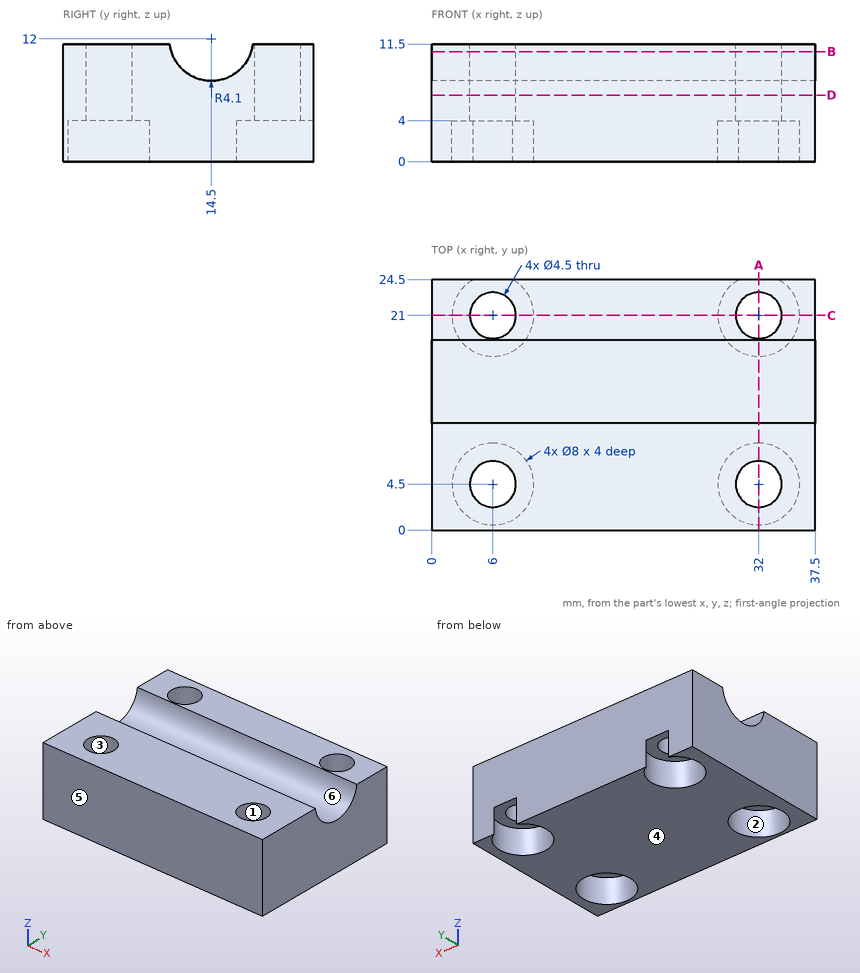
The drawing under review shows one solid part. Ordinate dimensions are in mm from its lowest x, y, z. A direction names the side the tool comes from. Round coordinates to 2 decimals unless told otherwise and drop trailing zeros. Order: outer loops, then holes, each group sorted by start corner. A loop starts at its lowest first (then second) coordinate and runs counter-clockwise, first axis right, second up. Notation, with made-up numbers: M -19,81.25 L -6,81.25 A26 cw -6,116.25 Z; hole C 3.25,12 d4. An arc over 180 degrees is marked long. Answer as CSV lines item,"result". Start each with the question number.
1) For pin 1 Ø3.5 at (x, y) = (6, 21) entering from +Z; pin 2 Ø4 at (x, y) = (6.5, 4) entering from -Z, all flat-tipped, find the tip position at first contact; note any pin that passes through.
2) Tool access review of the marked faces 1 and 2: name each direction out of +Z, -Z, +X, -X, +Y, -Y from which nothing blocks a thin tool from reaching the whole face with its end or side.
3) Add section C-C (y = 21). Give the boundary of the cut face in (x, z), then the cut area to 3 significant figures.
4) The part is to be moulded in two halves that separate along Y. For the marked faces 3, 4, 5 and 6, say which applies: +Y half, -Y half, draft (parallel to the pull), parting line (faces both ways), or undercut.
5) Wall thickness on line 1 along X through (y, z) = (4.5, 5.5); line 2 along X through (y, z) = (4.5, 2.8); line 3 along Y through (x, z) = (6, 8.5): over which ranges is each line inside the solid? List them lowest first. Write a range as [from, to].
6) Add section A-A (x = 32). Give the boundary of the cut face in (y, z), then the cut area to 3 significant figures.
7) Add section B-B (z = 10.75). Give the boundary of the cut face in (x, y).
8) Add section D-D (z = 6.5). Give the boundary of the cut face in (x, y), then the cut area to 3 significant figures.
Resolved:
1,pin 1,"through"
1,pin 2,"z = 4"
2,face 1,"+Z, -Z"
2,face 2,"-Z"
3,outline,"M 0,0 L 2,0 L 2,4 L 3.75,4 L 3.75,11.5 L 0,11.5 Z; M 8.25,4 L 10,4 L 10,0 L 28,0 L 28,4 L 29.75,4 L 29.75,11.5 L 8.25,11.5 Z; M 34.25,4 L 36,4 L 36,0 L 37.5,0 L 37.5,11.5 L 34.25,11.5 Z"
3,area,"300 mm^2"
4,face 3,"undercut"
4,face 4,"draft"
4,face 5,"-Y half"
4,face 6,"undercut"
5,line 1,"[0, 3.75], [8.25, 29.75], [34.25, 37.5]"
5,line 2,"[0, 2], [10, 28], [36, 37.5]"
5,line 3,"[0, 2.25], [6.75, 12.36], [16.64, 18.75], [23.25, 24.5]"
6,outline,"M 0,0 L 0.5,0 L 0.5,4 L 2.25,4 L 2.25,11.5 L 0,11.5 Z; M 6.75,4 L 8.5,4 L 8.5,0 L 17,0 L 17,4 L 18.75,4 L 18.75,11.5 L 18.57,11.5 A4.1 cw 10.43,11.5 L 6.75,11.5 Z; M 23.25,4 L 24.5,4 L 24.5,11.5 L 23.25,11.5 Z"
6,area,"130 mm^2"
7,outline,"M 0,0 L 37.5,0 L 37.5,10.6 L 0,10.6 Z; M 0,18.4 L 37.5,18.4 L 37.5,24.5 L 0,24.5 Z; hole C 6,4.5 d4.5; hole C 6,21 d4.5; hole C 32,4.5 d4.5; hole C 32,21 d4.5"
8,outline,"M 0,0 L 37.5,0 L 37.5,24.5 L 0,24.5 Z; hole C 6,4.5 d4.5; hole C 6,21 d4.5; hole C 32,4.5 d4.5; hole C 32,21 d4.5"
8,area,"855 mm^2"
